from build123d import *

# Parameters (mm, degrees)
SKETCH_1_W                   = 120
SKETCH_1_H                   = 100
EXTRUDE_1_DEPTH              = 7
SKETCH_2_R                   = 2.8
CUT_EXTRUDE_1_DEPTH          = 4
CUT_EXTRUDE_2_REACH          = 88.116
SKETCH_3_R                   = 1.6
SKETCH_4_W                   = 8
SKETCH_4_H                   = 100
EXTRUDE_2_DEPTH              = 10
HOLE_WIZARD_M3_5_D           = 2.5
HOLE_WIZARD_M3_5_CSINK_D     = 3.05
HOLE_WIZARD_M3_5_CSINK_ANGLE = 90


with BuildPart() as part:
    # 草图1 → 凸台-拉伸1 (new body)
    with BuildSketch(Plane(origin=(0, 0, 0), x_dir=(1, 0, 0), z_dir=(0, 1, 0))):
        with Locations((10, 0)):
            Rectangle(SKETCH_1_W, SKETCH_1_H)
    extrude(amount=EXTRUDE_1_DEPTH)

    # 草图2 → 切除-拉伸1 (cut)
    with BuildSketch(Plane.XZ):
        with Locations(Location((62, 38, 0), (0, 0, 270))):
            Circle(SKETCH_2_R)
        with Locations(Location((-30, 38, 0), (0, 0, 270))):
            Circle(SKETCH_2_R)
        with Locations(Location((-30, -14, 0), (0, 0, 270))):
            Circle(SKETCH_2_R)
        with Locations(Location((62, -14, 0), (0, 0, 270))):
            Circle(SKETCH_2_R)
        with Locations(Location((-20, 38, 0), (0, 0, 270))):
            Circle(SKETCH_2_R)
        with Locations(Location((50, 38, 0), (0, 0, 270))):
            Circle(SKETCH_2_R)
        with Locations(Location((50, -32, 0), (0, 0, 270))):
            Circle(SKETCH_2_R)
        with Locations(Location((-20, -32, 0), (0, 0, 270))):
            Circle(SKETCH_2_R)
    extrude(amount=-CUT_EXTRUDE_1_DEPTH, mode=Mode.SUBTRACT)

    # 草图3 → 切除-拉伸2 (cut, up to next)
    with BuildSketch(Plane.XZ.offset(-4), mode=Mode.PRIVATE) as cut_extrude_2_sk1:
        with Locations(Location((62, 38, 0), (0, 0, 270))):
            Circle(SKETCH_3_R)
    cut_extrude_2_tool1 = extrude(cut_extrude_2_sk1.sketch, amount=-CUT_EXTRUDE_2_REACH, mode=Mode.PRIVATE) & part.part
    # 草图3 → 切除-拉伸2 (cut, up to next)
    with BuildSketch(Plane.XZ.offset(-4), mode=Mode.PRIVATE) as cut_extrude_2_sk2:
        with Locations(Location((-30, 38, 0), (0, 0, 270))):
            Circle(SKETCH_3_R)
    cut_extrude_2_tool2 = extrude(cut_extrude_2_sk2.sketch, amount=-CUT_EXTRUDE_2_REACH, mode=Mode.PRIVATE) & part.part
    # 草图3 → 切除-拉伸2 (cut, up to next)
    with BuildSketch(Plane.XZ.offset(-4), mode=Mode.PRIVATE) as cut_extrude_2_sk3:
        with Locations(Location((-30, -14, 0), (0, 0, 270))):
            Circle(SKETCH_3_R)
    cut_extrude_2_tool3 = extrude(cut_extrude_2_sk3.sketch, amount=-CUT_EXTRUDE_2_REACH, mode=Mode.PRIVATE) & part.part
    # 草图3 → 切除-拉伸2 (cut, up to next)
    with BuildSketch(Plane.XZ.offset(-4), mode=Mode.PRIVATE) as cut_extrude_2_sk4:
        with Locations(Location((62, -14, 0), (0, 0, 270))):
            Circle(SKETCH_3_R)
    cut_extrude_2_tool4 = extrude(cut_extrude_2_sk4.sketch, amount=-CUT_EXTRUDE_2_REACH, mode=Mode.PRIVATE) & part.part
    # 草图3 → 切除-拉伸2 (cut, up to next)
    with BuildSketch(Plane.XZ.offset(-4), mode=Mode.PRIVATE) as cut_extrude_2_sk5:
        with Locations(Location((-20, 38, 0), (0, 0, 270))):
            Circle(SKETCH_3_R)
    cut_extrude_2_tool5 = extrude(cut_extrude_2_sk5.sketch, amount=-CUT_EXTRUDE_2_REACH, mode=Mode.PRIVATE) & part.part
    # 草图3 → 切除-拉伸2 (cut, up to next)
    with BuildSketch(Plane.XZ.offset(-4), mode=Mode.PRIVATE) as cut_extrude_2_sk6:
        with Locations(Location((50, 38, 0), (0, 0, 270))):
            Circle(SKETCH_3_R)
    cut_extrude_2_tool6 = extrude(cut_extrude_2_sk6.sketch, amount=-CUT_EXTRUDE_2_REACH, mode=Mode.PRIVATE) & part.part
    # 草图3 → 切除-拉伸2 (cut, up to next)
    with BuildSketch(Plane.XZ.offset(-4), mode=Mode.PRIVATE) as cut_extrude_2_sk7:
        with Locations(Location((50, -32, 0), (0, 0, 270))):
            Circle(SKETCH_3_R)
    cut_extrude_2_tool7 = extrude(cut_extrude_2_sk7.sketch, amount=-CUT_EXTRUDE_2_REACH, mode=Mode.PRIVATE) & part.part
    # 草图3 → 切除-拉伸2 (cut, up to next)
    with BuildSketch(Plane.XZ.offset(-4), mode=Mode.PRIVATE) as cut_extrude_2_sk8:
        with Locations(Location((-20, -32, 0), (0, 0, 270))):
            Circle(SKETCH_3_R)
    cut_extrude_2_tool8 = extrude(cut_extrude_2_sk8.sketch, amount=-CUT_EXTRUDE_2_REACH, mode=Mode.PRIVATE) & part.part
    add(cut_extrude_2_tool1.solids().sort_by_distance((62, 4, 38))[0], mode=Mode.SUBTRACT)
    add(cut_extrude_2_tool2.solids().sort_by_distance((-30, 4, 38))[0], mode=Mode.SUBTRACT)
    add(cut_extrude_2_tool3.solids().sort_by_distance((-30, 4, -14))[0], mode=Mode.SUBTRACT)
    add(cut_extrude_2_tool4.solids().sort_by_distance((62, 4, -14))[0], mode=Mode.SUBTRACT)
    add(cut_extrude_2_tool5.solids().sort_by_distance((-20, 4, 38))[0], mode=Mode.SUBTRACT)
    add(cut_extrude_2_tool6.solids().sort_by_distance((50, 4, 38))[0], mode=Mode.SUBTRACT)
    add(cut_extrude_2_tool7.solids().sort_by_distance((50, 4, -32))[0], mode=Mode.SUBTRACT)
    add(cut_extrude_2_tool8.solids().sort_by_distance((-20, 4, -32))[0], mode=Mode.SUBTRACT)

    # 草图4 → 凸台-拉伸2 (add)
    with BuildSketch(Plane.XZ):
        with Locations((-46, 0)):
            Rectangle(SKETCH_4_W, SKETCH_4_H)
        with Locations((24, 0)):
            Rectangle(SKETCH_4_W, SKETCH_4_H)
    extrude(amount=EXTRUDE_2_DEPTH)

    # M3 螺纹孔5 (through all)
    with Locations(Plane.XZ.offset(10)):
        with Locations((-46, -45), (24, -45), (24, 25), (-46, 25)):
            CounterSinkHole(HOLE_WIZARD_M3_5_D / 2, HOLE_WIZARD_M3_5_CSINK_D / 2, counter_sink_angle=HOLE_WIZARD_M3_5_CSINK_ANGLE)


solid = part.part
Build history of the part. All positions in model axes, mm. A direction names the side the tool comes from. Coordinates: 2 decimals unless noted, no trailing zeros. Write each loop counter-clockwise with the first axis right and the second up, starting at its lowest first coordinate (ties: lowest second). Pieces come first, ordered by that corner, then holes. Notation, with made-up numbers: (57, 9.25) -> (96, 9.25) arc R17 cw to (96, 24.25) -> close; hole circle Ø7 at (66, 30). An arc over 180 degrees is marked (long way). Use CSV: the item, a comma, the result in double quotes. Start each with the question number.
Q1. Cut at C-C, the plane z = -14. List the corners of the cut face in (x, y).
Q2. Drill centre lines: probe 1 along X at (y, z) = (5.25, -14); probe 2 along Z at (x, y) = (24, 1.25); probe 3 along X at (y, z) = (5.35, 38). Where is each one in solid material? Low to high.
Q3. Cut at B-B, the plane x = 50. List the corners of the cut face in (y, z).
Q4. Pull direction Z, two halves, no side cores. Call faces 4 (the flat face through (49, 0, -1)), 5 (the cylindrical face through (47.267, 1.972, 38.607)): released by +Z, released by -Z, zero draft, split by the parting line, or undercut.
Q5. Cut at D-D, the plane z = 1. List the corners of the cut face in (x, y).
Q6. 3-axis set-ups, long thin cutter, end or side, ignore diameter. For faces 1 (the flat face through (-11, 0, -1)), 2 (the flat face through (70, 3, 1)), 3 (the flat face through (62, 4, 36)): which of +Z, -Z, +X, -X, +Y, -Y reach the whole face in a straight line?
Q7. Flat gauge pins, fed straight in: pin 1 Ø3 at (x, z) = (49.5, -33) entering from -Y; pin 2 Ø3 at (y, z) = (-8.5, -34) entering from +X; pin 3 Ø21 at (x, z) = (52, -12) entering from -Y. Where does each tip first touch, or does it go through?
Q8. Cut at A-A, the plane y = -2.25. List the corners of the cut face in (x, z).
Checked values:
1,outline,"(-50, -10) -> (-42, -10) -> (-42, 0) -> (-32.8, 0) -> (-32.8, 4) -> (-31.6, 4) -> (-31.6, 7) -> (-50, 7) -> close; (-28.4, 4) -> (-27.2, 4) -> (-27.2, 0) -> (20, 0) -> (20, -10) -> (28, -10) -> (28, 0) -> (59.2, 0) -> (59.2, 4) -> (60.4, 4) -> (60.4, 7) -> (-28.4, 7) -> close; (63.6, 4) -> (64.8, 4) -> (64.8, 0) -> (70, 0) -> (70, 7) -> (63.6, 7) -> close"
2,probe 1,"x = -50 to -31.6, -28.4 to 60.4, 63.6 to 70"
2,probe 2,"z = -50 to -46.25, -43.75 to 23.75, 26.25 to 50"
2,probe 3,"x = -50 to -31.6, -28.4 to -21.6, -18.4 to 48.4, 51.6 to 60.4, 63.6 to 70"
3,outline,"(0, -50) -> (7, -50) -> (7, -33.6) -> (4, -33.6) -> (4, -34.8) -> (0, -34.8) -> close; (0, -29.2) -> (4, -29.2) -> (4, -30.4) -> (7, -30.4) -> (7, 36.4) -> (4, 36.4) -> (4, 35.2) -> (0, 35.2) -> close; (0, 40.8) -> (4, 40.8) -> (4, 39.6) -> (7, 39.6) -> (7, 50) -> (0, 50) -> close"
4,face 4,"zero draft"
4,face 5,"undercut"
5,outline,"(-50, -10) -> (-42, -10) -> (-42, 0) -> (20, 0) -> (20, -10) -> (28, -10) -> (28, 0) -> (70, 0) -> (70, 7) -> (-50, 7) -> close"
6,face 1,"+Z, -Z, -Y"
6,face 2,"+Z, -Z, +X, +Y, -Y"
6,face 3,"-Y"
7,pin 1,"stops at y = 4"
7,pin 2,"stops at x = 28"
7,pin 3,"stops at y = 0"
8,outline,"(-50, -50) -> (-42, -50) -> (-42, 50) -> (-50, 50) -> close; (20, -50) -> (28, -50) -> (28, 50) -> (20, 50) -> close; hole circle Ø2.5 at (-46, -45); hole circle Ø2.5 at (-46, 25); hole circle Ø2.5 at (24, -45); hole circle Ø2.5 at (24, 25)"
